```python
from build123d import *

# Parameters (mm, degrees)
SKETCH1_R           = 30
BOSS_EXTRUDE1_DEPTH = 10
BOSS_EXTRUDE2_DEPTH = 20
SKETCH3_R           = 20
BOSS_EXTRUDE3_DEPTH = 50
CUT_EXTRUDE1_DEPTH  = 10
SKETCH5_R           = 15
CUT_EXTRUDE2_DEPTH  = 41
SKETCH6_R           = 8
CUT_EXTRUDE3_DEPTH  = 91


with BuildPart() as part:
    # Sketch1 → Boss-Extrude1 (new body, symmetric)
    with BuildSketch(Plane(origin=(0, 0, 0), x_dir=(0, 0, -1), z_dir=(1, 0, 0))):
        Circle(SKETCH1_R)
    extrude(amount=BOSS_EXTRUDE1_DEPTH, both=True)

    # Sketch2 → Boss-Extrude2 (add)
    with BuildSketch(Plane(origin=(10, 0, 0), x_dir=(0, 0, -1), z_dir=(1, 0, 0))):
        with BuildLine():
            ThreePointArc((36.043181696, -17.346153846), (0, 40), (-36.043181696, -17.346153846))
            ThreePointArc((-36.043181696, -17.346153846), (-27.235626529, -52.234661385), (-32.799295343, -87.785))
            ThreePointArc((-32.799295343, -87.785), (0, -135), (32.799295343, -87.785))
            ThreePointArc((32.799295343, -87.785), (27.235626529, -52.234661385), (36.043181696, -17.346153846))
        make_face()
    boss_extrude2 = extrude(amount=BOSS_EXTRUDE2_DEPTH)

    # Sketch3 → Boss-Extrude3 (add)
    with BuildSketch(Plane(origin=(30, 0, 0), x_dir=(0, 0, -1), z_dir=(1, 0, 0))):
        with Locations((0, -100)):
            Circle(SKETCH3_R)
    boss_extrude3 = extrude(amount=BOSS_EXTRUDE3_DEPTH)

    # Sketch4 → Cut-Extrude1 (cut)
    with BuildSketch(Plane(origin=(30, 0, 0), x_dir=(0, 0, -1), z_dir=(1, 0, 0))):
        with BuildLine():
            ThreePointArc((30.176724251, 7.096852363), (22.585383623, 21.234416559), (8.942307692, 29.682235986))
            ThreePointArc((8.942307692, 29.682235986), (2.712542583, 26.337086261), (6.057692308, 20.107321152))
            ThreePointArc((6.057692308, 20.107321152), (15.299776003, 14.384604766), (20.442297073, 4.807545149))
            ThreePointArc((20.442297073, 4.807545149), (26.454164269, 1.084985167), (30.176724251, 7.096852363))
        make_face()
        with BuildLine():
            ThreePointArc((-30.176724251, 7.096852363), (-22.585383623, 21.234416559), (-8.942307692, 29.682235986))
            ThreePointArc((-8.942307692, 29.682235986), (-2.712542583, 26.337086261), (-6.057692308, 20.107321152))
            ThreePointArc((-6.057692308, 20.107321152), (-15.299776003, 14.384604766), (-20.442297073, 4.807545149))
            ThreePointArc((-20.442297073, 4.807545149), (-26.454164269, 1.084985167), (-30.176724251, 7.096852363))
        make_face()
        with BuildLine():
            ThreePointArc((27.032386272, -13.009615385), (17.862474513, -44.37894553), (19.296651575, -77.029600831))
            ThreePointArc((19.296651575, -77.029600831), (0, -70), (-19.296651575, -77.029600831))
            ThreePointArc((-19.296651575, -77.029600831), (-17.862474513, -44.37894553), (-27.032386272, -13.009615385))
            ThreePointArc((-27.032386272, -13.009615385), (-24.695257791, -6.335948442), (-18.021590848, -8.673076923))
            ThreePointArc((-18.021590848, -8.673076923), (0, -20), (18.021590848, -8.673076923))
            ThreePointArc((18.021590848, -8.673076923), (24.695257791, -6.335948442), (27.032386272, -13.009615385))
        make_face()
    cut_extrude1 = extrude(amount=-CUT_EXTRUDE1_DEPTH, mode=Mode.SUBTRACT)

    # Sketch5 → Cut-Extrude2 (cut, through all)
    with BuildSketch(Plane(origin=(30, 0, 0), x_dir=(0, 0, -1), z_dir=(1, 0, 0))):
        Circle(SKETCH5_R)
    cut_extrude2 = extrude(amount=-CUT_EXTRUDE2_DEPTH, mode=Mode.SUBTRACT)

    # Sketch6 → Cut-Extrude3 (cut, through all)
    with BuildSketch(Plane(origin=(80, 0, 0), x_dir=(0, 0, -1), z_dir=(1, 0, 0))):
        with Locations((0, -100)):
            Circle(SKETCH6_R)
    cut_extrude3 = extrude(amount=-CUT_EXTRUDE3_DEPTH, mode=Mode.SUBTRACT)

    # Mirror1: Boss-Extrude2, Boss-Extrude3, Cut-Extrude1, Cut-Extrude2, Cut-Extrude3 across plane
    add(boss_extrude2.mirror(Plane(origin=(0, 0, 0), x_dir=(0, 0, 1), z_dir=(1, 0, 0))))
    add(boss_extrude3.mirror(Plane(origin=(0, 0, 0), x_dir=(0, 0, 1), z_dir=(1, 0, 0))))
    add(cut_extrude1.mirror(Plane(origin=(0, 0, 0), x_dir=(0, 0, 1), z_dir=(1, 0, 0))), mode=Mode.SUBTRACT)
    add(cut_extrude2.mirror(Plane(origin=(0, 0, 0), x_dir=(0, 0, 1), z_dir=(1, 0, 0))), mode=Mode.SUBTRACT)
    add(cut_extrude3.mirror(Plane(origin=(0, 0, 0), x_dir=(0, 0, 1), z_dir=(1, 0, 0))), mode=Mode.SUBTRACT)


solid = part.part
```
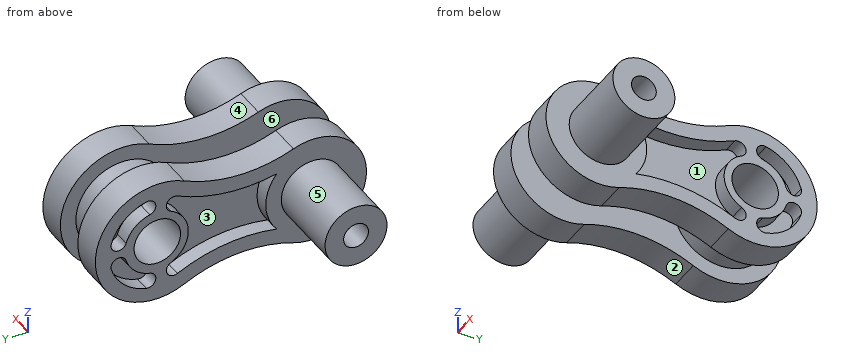
Could you check a few things on this model? Use its own coordinates, in mm. Face numbers are marked on the shaded views. A direction names the side the tool comes from. Round coordinates to 2 decimals unless told otherwise and drop trailing zeros. Loops run counter-clockwise (first coordinate to the right, second up) from the corner with the lowest first, then second, coordinate; pieces in that order, holes last.
Q1. Please list where these lines run through material, in increasing order: L1, parallel to X at y = -29, z = -13.5; L2, parallel to Y at x = -63.5, z = 0.5; L3, parallel to X at y = -124.5, z = 9.5.
Q2. On a 3-axis mill with a long thin cutter (end or side, diameter ignored), from which of +Z, -Z, +X, -X, +Y, -Y can I reach the whole of each face in a straight line? I mean the marked faces 1, 2 and 3. Say none if no direction works.
Q3. For P1, Ø3, axis at x = -26.5, z = -5, coming from the +Y side; P2, Ø24, axis at y = -16, z = 1.5, coming from the +X side; P3, Ø1, axis at x = 61, y = -104.5, coming from the -Z side, each with a flat end and sliding along its axis, tell me the tip position at first contact or that it passes through.
Q4. I want a section at A-A (y = -64). Write out the boundary of the cut face in (x, z), and give its area (3 significant figures).
Q5. I want a section at D-D (x = -39). Write out the boundary of the cut face in (y, z), and give its area (3 significant figures).
Q6. Thinking about a two-plate mould opening in Y: for the marked faces 4, 5 and 6, which applies, pulls with the +Y half, pulls with the -Y half, needs draft (parallel to the pull), parting line crosses it, or undercut?
Q7. I want a section at C-C (z = 0). Give the number of separate pieces and of enclosed holes in the cut face, and give its area (3 significant figures).
Q8. I want a section at B-B (x = -22.5). Write out the boundary of the cut face in (y, z) (3 decimals), and give its area (3 significant figures).
Answer below:
1. L1: x = -20 to -10, 10 to 20
1. L2: y = -119.99 to -107.98, -92.02 to -80.01
1. L3: x = -30 to -10, 10 to 30
2. face 1: +X
2. face 2: -Z, +X, -X
2. face 3: -X
3. P1: stops at y = 39.85
3. P2: stops at x = 30
3. P3: stops at z = -19.6
4. outline: (-30, -27.46) - (-10, -27.46) - (-10, 27.46) - (-30, 27.46) - (-30, 17.43) - (-20, 17.43) - (-20, -17.43) - (-30, -17.43) - close; (10, -27.46) - (30, -27.46) - (30, -17.43) - (20, -17.43) - (20, 17.43) - (30, 17.43) - (30, 27.46) - (10, 27.46) - close
4. area: 1,500 mm2
5. outline: circle Ø40 at (-100, 0); hole circle Ø16 at (-100, 0)
5. area: 1,060 mm2
6. face 4: undercut
6. face 5: parting line crosses it
6. face 6: needs draft
7. separate pieces: 4
7. enclosed holes: 0
7. area: 7,160 mm2
8. outline: (-87.785, -32.799) arc R90 cw to (-17.346, -36.043) arc R40 ccw (long way) to (-17.346, 36.043) arc R90 cw to (-87.785, 32.799) arc R35 ccw (long way) to start; hole circle Ø16 at (-100, 0); hole (-77.03, -19.297) arc R100 cw to (-13.01, -27.032) arc R5 ccw to (-8.673, -18.022) arc R20 cw to (-8.673, 18.022) arc R5 ccw to (-13.01, 27.032) arc R100 cw to (-77.03, 19.297) arc R30 cw to start; hole circle Ø30 at (0, 0); hole (4.808, -20.442) arc R5 ccw to (7.097, -30.177) arc R31 ccw to (29.682, -8.942) arc R5 ccw to (20.107, -6.058) arc R21 cw to start; hole (4.808, 20.442) arc R21 cw to (20.107, 6.058) arc R5 ccw to (29.682, 8.942) arc R31 ccw to (7.097, 30.177) arc R5 ccw to start
8. area: 6,880 mm2
